Autodesk Inventor part; units mm, degrees
ref_plane "YZ Plane" through (0, 0, 0) normal (1, 0, 0) x (0, 1, 0)
ref_plane "XZ Plane" through (0, 0, 0) normal (0, 1, 0) x (-1, 0, 0)
ref_plane "XY Plane" through (0, 0, 0) normal (0, 0, 1) x (1, 0, 0)
sketch "Sketch1" plane through (0, 0, 0) normal (0, 1, 0) x (-1, 0, 0)
  arc A0 (-7.3333, 0) -> (-10.6667, -3.3333) centre (-7.3333, -3.3333) ccw
  arc A1 (-7.3333, 0) -> (-7.3667, -0.0002) centre (-7.3333, -3.3333) ccw
  line L0 (-5.4282, -5.2385) -> (-8.0307, -5.9358)
  line L1 (-8.0307, -5.9358) -> (-5.4282, -5.2385)
  line L2 (-8.0307, -5.9358) -> (-9.9358, -4.0307)
  line L3 (-6.636, -0.7308) -> (-4.7308, -2.636)
  line L4 (-4.7308, -2.636) -> (-5.4282, -5.2385)
  line L5 (-8.0307, -5.9358) -> (-9.9358, -4.0307)
  line L6 (-6.636, -0.7308) -> (-4.7308, -2.636)
  line L7 (-6.636, -0.7308) -> (-7.3667, -0.0002)
  line L8 (-9.9358, -4.0307) -> (-10.6665, -3.3)
  arc A2 (-10.6665, -3.3) -> (-10.6667, -3.3333) centre (-7.3333, -3.3333) ccw
  arc A3 (-7.3667, -0.0002) -> (-10.6665, -3.3) centre (-7.3333, -3.3333) ccw construction
  circle A4 centre (-7.3333, -3.3333) radius 2
  point P0 (0, 0)
  dimension "d2" = 4
extrude "Extrusion1" add sketch "Sketch1" along normal blind 5
properties part number "NutInserperFilling" material "Nylon 6/6"
The model under review builds one solid part; all positions refer to its coordinate system, in mm. Coordinates: 2 decimals unless noted, no trailing zeros. Write each loop counter-clockwise with the first axis right and the second up, starting at its lowest first coordinate (ties: lowest second). Pieces come first, ordered by that corner, then holes. Notation, with made-up numbers: (-27, 9.25) - (-16, 9.25) arc R19 cw to (-16, 34.25) - close; hole circle Ø6 at (62, 53.25). An arc over 180 degrees is marked (long way). Answer in a Markdown table with one row per item. Add a question column.
Q1. Consider section A-A on x = 6.1. Give the boundary of the cut face in (y, z).
Q2. Consider section B-B on z = -3.8. Give the boundary of the cut face in (x, y).
Q3. Clearance check with flat-ended pins moving along their axes: pin 1 (1.5 mm diameter, centred on x = 5.5, y = 4.5, fed in from -Z); pin 2 (3 mm diameter, centred on x = 7, z = -2, fed in from -Y); pin 3 (3 mm diameter, centred on x = 5.5, y = 3, fed in from -Z); pin 4 (1.5 mm diameter, centred on x = 9.5, y = 3.5, fed in from -Z). State where each tip first meets the part, or that it passes through.
Q4. Draft analysis for pull direction X (two halves, no side actions). For faces 1 (the face through (9.3, 5, -2.3)), 2 (the face through (9.33, 2.465, -4.636)), 3 (the face through (6.26, 2.46, -5.02)), 4 (the face through (6.71, 2.46, -5.58)), state which applies: +X half, -X half, draft (parallel to the pull), parting line (faces both ways), or undercut.
Q5. To check wall thickness, follow line 1 along X through (y, z) = (3.65, -2.1); line 2 along Z through (x, y) = (6.1, 2.85); line 3 along Z through (x, y) = (8.2, 3.4). State the ranges of each line that lie inside material, in increasing order. Write a range as from..to.
Q6. Consider section D-D on z = -1. Give the boundary of the cut face in (x, y).
Q7. Consider section C-C on y = 0.65. Give the boundary of the cut face in (x, z).
Answers below:
| question | item | result |
|---|---|---|
| 1 | outline | (0, -5.42) - (5, -5.42) - (5, -4.91) - (0, -4.91) - close; (0, -1.76) - (5, -1.76) - (5, -1.27) - (0, -1.27) - close |
| 2 | outline | (5.04, 0) - (5.39, 0) - (5.39, 5) - (5.04, 5) - close; (9.28, 0) - (10.17, 0) - (10.17, 5) - (9.28, 5) - close |
| 3 | pin 1 | z = -5.46 |
| 3 | pin 2 | y = 0 |
| 3 | pin 3 | z = -5.66 |
| 3 | pin 4 | z = -5.22 |
| 4 | face 1 | draft |
| 4 | face 2 | +X half |
| 4 | face 3 | undercut |
| 4 | face 4 | -X half |
| 5 | line 1 | 5.27..5.76, 8.91..10.43 |
| 5 | line 2 | -5.42..-4.91, -1.76..-1.27 |
| 5 | line 3 | -5.77..-5.14, -1.53..-0.11 |
| 6 | outline | (6.37, 0) - (9.71, 0) - (9.71, 5) - (6.37, 5) - close |
| 7 | outline | (4.73, -2.64) - (5.43, -5.24) - (8.03, -5.94) - (10.67, -3.3) arc R3.33 ccw to (7.37, 0) - (6.64, -0.73) - close; hole circle Ø4 at (7.33, -3.33) |
